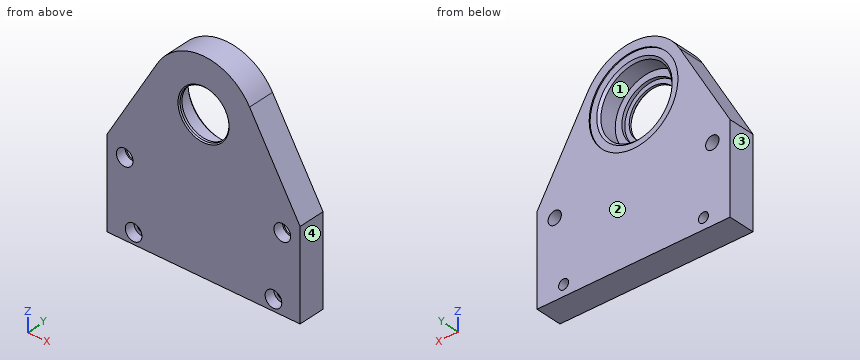
from build123d import *

# Parameters (mm, degrees)
F0_R     = 11
F1_DEPTH = 12
F2_R     = 3
F3_DEPTH = 18
F2_R_2   = 3.75
F4_DEPTH = 4.5
F2_R_3   = 2.25
F5_DEPTH = 12.001
F6_DEPTH = 4.5
F10_SIZE = 0.5


# Not quite as in the source:
# - a pattern or mirror of a feature is missing from the dataset's text; its kind, count and spacing are read off the source's solid


with BuildPart() as f1:
    # F0 (on Front) → F1 (new body)
    with BuildSketch(Plane.XZ):
        with BuildLine():
            Line((-43.5, 40), (-43.5, 0))
            Line((-43.5, 0), (43.5, 0))
            Line((43.5, 0), (43.5, 40))
            Line((43.5, 40), (20.7387457553, 79.0790903836))
            ThreePointArc((20.7387457553, 79.0790903836), (0, 91), (-20.7387457553, 79.0790903836))
            Line((-20.7387457553, 79.0790903836), (-43.5, 40))
        make_face()
        with Locations((0, 67)):
            Circle(F0_R, mode=Mode.SUBTRACT)
    extrude(amount=F1_DEPTH)

    # F2 (on face) → F3 (cut)
    with BuildSketch(Plane.XZ.offset(12)):
        with Locations((-35.5, 34)):
            Circle(F2_R)
    f3 = extrude(amount=-F3_DEPTH, mode=Mode.SUBTRACT)

    # F3_copies: F3 across plane
    add(f3.mirror(Plane(origin=(0, 0, 0), x_dir=(0, 0, 1), z_dir=(1, 0, 0))), mode=Mode.SUBTRACT)

    # F2 (on face) → F4 (cut)
    with BuildSketch(Plane.XZ.offset(12)):
        with Locations((-35.5, 34)):
            Circle(F2_R_2)
        with Locations((-35.5, 34)):
            Circle(F2_R, mode=Mode.SUBTRACT)
    f4 = extrude(amount=-F4_DEPTH, mode=Mode.SUBTRACT)

    # F4_copies: F4 across plane
    add(f4.mirror(Plane(origin=(0, 0, 0), x_dir=(0, 0, 1), z_dir=(1, 0, 0))), mode=Mode.SUBTRACT)

    # F2 (on face) → F5 (cut, through all)
    with BuildSketch(Plane.XZ.offset(12)):
        with Locations((-31.5, 5)):
            Circle(F2_R_3)
    f5 = extrude(amount=-F5_DEPTH, mode=Mode.SUBTRACT)

    # F5_copies: F5 across plane
    add(f5.mirror(Plane(origin=(0, 0, 0), x_dir=(0, 0, 1), z_dir=(1, 0, 0))), mode=Mode.SUBTRACT)

    # F2 (on face) → F6 (cut)
    with BuildSketch(Plane.XZ.offset(12)):
        with Locations((-31.5, 5)):
            Circle(F2_R_2)
        with Locations((-31.5, 5)):
            Circle(F2_R_3, mode=Mode.SUBTRACT)
    f6 = extrude(amount=-F6_DEPTH, mode=Mode.SUBTRACT)

    # F6_copies: F6 across plane
    add(f6.mirror(Plane(origin=(0, 0, 0), x_dir=(0, 0, 1), z_dir=(1, 0, 0))), mode=Mode.SUBTRACT)

    # F8 (on offset) → F9 (revolve, cut)
    with BuildSketch(Plane.XY.offset(67)):
        Polygon((0, 0), (0, -12), (11, -12), (11, -10.5), (13, -10.5), (13, -9), (16, -9), (16, -1.5), (17, -0.5), (20, -0.5), (20, 0), align=None)
    revolve(axis=Axis((0, -9.5826864708, 67), (0, 1, 0)), mode=Mode.SUBTRACT)

    # F10
    f10_edges = [f1.edges().sort_by_distance(p)[0] for p in [
        (-11, -12, 67),
    ]]
    chamfer(f10_edges, length=F10_SIZE)


solid = f1.part
Read the model definition and answer for the solid it produces. Units are mm, in the model's axes. Face numbers are marked on the shaded views. Give positions to 0.01 mm unless a question says otherwise; leave off trailing zeros. Write each loop counter-clockwise with the first axis right and the second up, starting at its lowest first coordinate (ties: lowest second). Pieces come first, ordered by that corner, then holes. Notation, with made-up numbers: (1, 26.5) -> (46, 26.5) arc R25 cw to (46, 43.5) -> close; hole circle Ø4 at (-28, 32). An arc over 180 degrees is marked (long way). Answer as a JSON object with one key per item and string values. Group by question number.
1) Find section A-A (x = 0). Write down the section's boundary in (y, z), and give its area (3 significant figures).
2) Find section D-D (z = 67). Write down the section's boundary in (x, y), and give its area (3 significant figures).
3) Find section B-B (z = 5). Write down the section's boundary in (x, y).
4) Find section C-C (y = -4.5). Write down the section's boundary in (x, z), and give its area (3 significant figures).
5) Consider L1, parallel to X at y = -0.25, z = 67; L2, parallel to X at y = -7.75, z = 67; L3, parallel to Y at x = 9, z = 57. Determine where each line is inside the solid, lowest interval first. Write a range as from..to.
6) The mould has two halves that part along X. Classify the marked faces 1, 2, 3 and 4: +X half, -X half, draft (parallel to the pull), parting line (faces both ways), or undercut.
7) Each of these flat-tipped pins is pushed along its axis until it touches: P1, Ø3, axis at x = 25, y = -9, coming from the +Z side; P2, Ø21, axis at x = 2, z = 63, coming from the +Y side; P3, Ø6, axis at x = 31.5, z = 5, coming from the -Y side. Where does it stop, or does it pass through?
Values follow:
{
 "1": {"outline": "(-12, 0) -> (0, 0) -> (0, 47) -> (-0.5, 47) -> (-0.5, 50) -> (-1.5, 51) -> (-9, 51) -> (-9, 54) -> (-10.5, 54) -> (-10.5, 56) -> (-11.5, 56) -> (-12, 55.5) -> close; (-12, 78.5) -> (-11.5, 78) -> (-10.5, 78) -> (-10.5, 80) -> (-9, 80) -> (-9, 83) -> (-1.5, 83) -> (-0.5, 84) -> (-0.5, 87) -> (0, 87) -> (0, 91) -> (-12, 91) -> close", "area": "727 mm2"},
 "2": {"outline": "(-27.77, -12) -> (-11.5, -12) -> (-11, -11.5) -> (-11, -10.5) -> (-13, -10.5) -> (-13, -9) -> (-16, -9) -> (-16, -1.5) -> (-17, -0.5) -> (-20, -0.5) -> (-20, 0) -> (-27.77, 0) -> close; (11, -11.5) -> (11.5, -12) -> (27.77, -12) -> (27.77, 0) -> (20, 0) -> (20, -0.5) -> (17, -0.5) -> (16, -1.5) -> (16, -9) -> (13, -9) -> (13, -10.5) -> (11, -10.5) -> close", "area": "301 mm2"},
 "3": {"outline": "(-43.5, -12) -> (-35.25, -12) -> (-35.25, -7.5) -> (-33.75, -7.5) -> (-33.75, 0) -> (-43.5, 0) -> close; (-29.25, -7.5) -> (-27.75, -7.5) -> (-27.75, -12) -> (27.75, -12) -> (27.75, -7.5) -> (29.25, -7.5) -> (29.25, 0) -> (-29.25, 0) -> close; (33.75, -7.5) -> (35.25, -7.5) -> (35.25, -12) -> (43.5, -12) -> (43.5, 0) -> (33.75, 0) -> close"},
 "4": {"outline": "(-43.5, 0) -> (43.5, 0) -> (43.5, 40) -> (20.74, 79.08) arc R24 ccw to (-20.74, 79.08) -> (-43.5, 40) -> close; hole circle Ø6 at (-35.5, 34); hole circle Ø4.5 at (-31.5, 5); hole circle Ø32 at (0, 67); hole circle Ø4.5 at (31.5, 5); hole circle Ø6 at (35.5, 34)", "area": "5,450 mm2"},
 "5": {"L1": "x = -27.77..-20, 20..27.77", "L2": "x = -27.77..-16, 16..27.77", "L3": "y = -12..-9"},
 "6": {"face 1": "undercut", "face 2": "draft", "face 3": "-X half", "face 4": "+X half"},
 "7": {"P1": "stops at z = 74.34", "P2": "stops at y = -9", "P3": "stops at y = -7.5"}
}
